Build history of the part. All positions in model axes, mm. Round coordinates to 2 decimals unless told otherwise and drop trailing zeros. Order: outer loops, then holes, each group sorted by start corner. A loop starts at its lowest first (then second) coordinate and runs counter-clockwise, first axis right, second up. Notation, with made-up numbers: (86, -35.75) - (141, -35.75) arc R33 cw to (141, -6.75) - close; hole circle Ø3 at (51, 17). An arc over 180 degrees is marked (long way). Write each question's results on one line, items separated by ' | '. Start each with the question number.
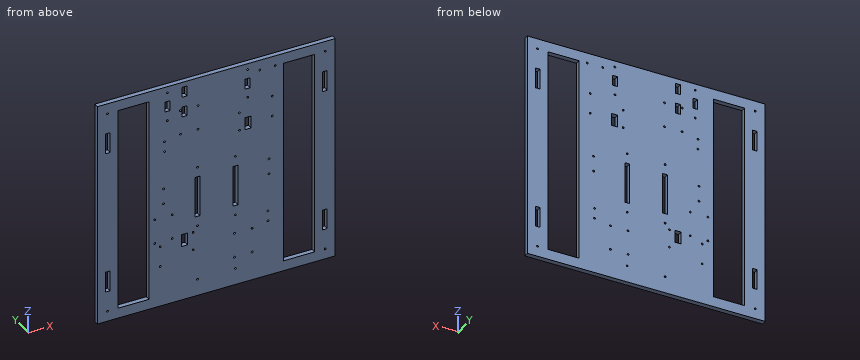
```python
from build123d import *

# Parameters (mm, degrees)
SKETCH1_W           = 292.1
SKETCH1_H           = 279.4
BOSS_EXTRUDE1_DEPTH = 5.9436
SKETCH2_W           = 38.1
SKETCH2_H           = 254
SKETCH2_W_2         = 5.9309
SKETCH2_H_2         = 25.4
CUT_EXTRUDE1_DEPTH  = 6.9436
SKETCH5_R           = 1.1303
SKETCH5_W           = 7.366
SKETCH5_H           = 15.24
CUT_EXTRUDE2_DEPTH  = 6.9436
SKETCH7_R           = 1.1303
SKETCH7_W           = 5.9436
SKETCH7_H           = 12.7
CUT_EXTRUDE3_DEPTH  = 6.9436
SKETCH9_R           = 1.1303
CUT_EXTRUDE4_DEPTH  = 6.9436
SKETCH10_W          = 5.9436
SKETCH10_H          = 50.8
CUT_EXTRUDE5_DEPTH  = 6.9436
SKETCH12_R          = 1.1303
CUT_EXTRUDE6_DEPTH  = 6.9436


with BuildPart() as part:
    # Sketch1 → Boss-Extrude1 (new body)
    with BuildSketch(Plane(origin=(0, 0, 0), x_dir=(1, 0, 0), z_dir=(0, 1, 0))):
        Rectangle(SKETCH1_W, SKETCH1_H)
    extrude(amount=BOSS_EXTRUDE1_DEPTH)

    # Sketch2 → Cut-Extrude1 (cut, through all)
    with BuildSketch(Plane(origin=(0, 5.9436, 0), x_dir=(1, 0, 0), z_dir=(0, 1, 0))):
        with Locations((-101.6, 0)):
            Rectangle(SKETCH2_W, SKETCH2_H)
        with Locations((101.6, 0)):
            Rectangle(SKETCH2_W, SKETCH2_H)
        with Locations((133.35, 88.9)):
            Rectangle(SKETCH2_W_2, SKETCH2_H_2)
        with Locations((-133.35, 88.9)):
            Rectangle(SKETCH2_W_2, SKETCH2_H_2)
        with Locations((133.35, -88.9)):
            Rectangle(SKETCH2_W_2, SKETCH2_H_2)
        with Locations((-133.35, -88.9)):
            Rectangle(SKETCH2_W_2, SKETCH2_H_2)
    extrude(amount=-CUT_EXTRUDE1_DEPTH, mode=Mode.SUBTRACT)

    # Sketch5 → Cut-Extrude2 (cut, through all)
    with BuildSketch(Plane.XZ):
        with Locations((-43.99385, 104.14)):
            Circle(SKETCH5_R)
        with Locations((-22.40385, 104.14)):
            Circle(SKETCH5_R)
        with Locations((-43.99385, 73.66)):
            Circle(SKETCH5_R)
        with Locations((-22.40385, 73.66)):
            Circle(SKETCH5_R)
        with Locations((28.37815, 79.502)):
            Circle(SKETCH5_R)
        with Locations((28.37815, 57.15)):
            Circle(SKETCH5_R)
        with Locations((68.761578288, 88.9)):
            Circle(SKETCH5_R)
        with Locations((68.761578288, 63.5)):
            Circle(SKETCH5_R)
        with Locations((-63.5, 69.85)):
            Circle(SKETCH5_R)
        with Locations((44.00655, -73.66)):
            Circle(SKETCH5_R)
        with Locations((44.00655, -104.14)):
            Circle(SKETCH5_R)
        with Locations((22.41655, -104.14)):
            Circle(SKETCH5_R)
        with Locations((22.41655, -73.66)):
            Circle(SKETCH5_R)
        with Locations((-28.36545, -79.502)):
            Circle(SKETCH5_R)
        with Locations((-28.36545, -57.15)):
            Circle(SKETCH5_R)
        with Locations((-68.748878288, -63.5)):
            Circle(SKETCH5_R)
        with Locations((-68.748878288, -88.9)):
            Circle(SKETCH5_R)
        with Locations((-63.5, 57.15)):
            Circle(SKETCH5_R)
        with Locations((63.5, -69.85)):
            Circle(SKETCH5_R)
        with Locations((63.5, -57.15)):
            Circle(SKETCH5_R)
        with Locations((-64.77, 9.627315903)):
            Circle(SKETCH5_R)
        with Locations((-64.77, -9.422684097)):
            Circle(SKETCH5_R)
        with Locations((64.77, -9.610296009)):
            Circle(SKETCH5_R)
        with Locations((64.77, 9.439703991)):
            Circle(SKETCH5_R)
        with Locations((-133.7564, -127)):
            Circle(SKETCH5_R)
        with Locations((-133.7564, 127)):
            Circle(SKETCH5_R)
        with Locations((133.7564, -127)):
            Circle(SKETCH5_R)
        with Locations((133.7564, 127)):
            Circle(SKETCH5_R)
        with Locations((39.17315, 63.5)):
            Rectangle(SKETCH5_W, SKETCH5_H)
        with Locations((-39.16045, -63.5)):
            Rectangle(SKETCH5_W, SKETCH5_H)
    extrude(amount=-CUT_EXTRUDE2_DEPTH, mode=Mode.SUBTRACT)

    # Sketch7 → Cut-Extrude3 (cut, through all)
    with BuildSketch(Plane(origin=(0, 5.9436, 0), x_dir=(1, 0, 0), z_dir=(0, 1, 0))):
        with Locations((53.410346989, -127)):
            Circle(SKETCH7_R)
        with Locations((72.460346989, -127)):
            Circle(SKETCH7_R)
        with Locations((-60.069552222, -95.996553949)):
            Circle(SKETCH7_R)
        with Locations((-60.069552222, -131.742630767)):
            Circle(SKETCH7_R)
        with Locations((38.527322113, -96.482293749)):
            Circle(SKETCH7_R)
        with Locations((38.527322113, -132.062224084)):
            Circle(SKETCH7_R)
        with Locations((-60.059259893, -114.3)):
            Rectangle(SKETCH7_W, SKETCH7_H)
        with Locations((-38.875659893, -101.6)):
            Rectangle(SKETCH7_W, SKETCH7_H)
        with Locations((-38.875659893, -127)):
            Rectangle(SKETCH7_W, SKETCH7_H)
        with Locations((38.527322113, -114.207868653)):
            Rectangle(SKETCH7_W, SKETCH7_H)
    extrude(amount=-CUT_EXTRUDE3_DEPTH, mode=Mode.SUBTRACT)

    # Sketch9 → Cut-Extrude4 (cut, through all)
    with BuildSketch(Plane(origin=(0, 5.9436, 0), x_dir=(1, 0, 0), z_dir=(0, 1, 0))):
        with Locations((23.4442, 50.154484486)):
            Circle(SKETCH9_R)
        with Locations((23.4442, 119.039284486)):
            Circle(SKETCH9_R)
        with Locations((23.4442, -25.086665514)):
            Circle(SKETCH9_R)
        with Locations((-23.1394, 119.039284486)):
            Circle(SKETCH9_R)
        with Locations((-23.1394, 50.154484486)):
            Circle(SKETCH9_R)
        with Locations((-23.1394, -25.086665514)):
            Circle(SKETCH9_R)
    extrude(amount=-CUT_EXTRUDE4_DEPTH, mode=Mode.SUBTRACT)

    # Sketch10 → Cut-Extrude5 (cut, through all)
    with BuildSketch(Plane(origin=(0, 5.9436, 0), x_dir=(1, 0, 0), z_dir=(0, 1, 0))):
        with Locations((23.4442, 12.665075)):
            Rectangle(SKETCH10_W, SKETCH10_H)
        with Locations((-23.1394, 12.665075)):
            Rectangle(SKETCH10_W, SKETCH10_H)
    extrude(amount=-CUT_EXTRUDE5_DEPTH, mode=Mode.SUBTRACT)

    # Sketch12 → Cut-Extrude6 (cut, through all)
    with BuildSketch(Plane(origin=(0, 5.9436, 0), x_dir=(1, 0, 0), z_dir=(0, 1, 0))):
        with Locations((-75.6666, 26.7462)):
            Circle(SKETCH12_R)
        with Locations((-75.6666, 57.2262)):
            Circle(SKETCH12_R)
        with Locations((-54.0766, 57.2262)):
            Circle(SKETCH12_R)
        with Locations((-54.0766, 26.7462)):
            Circle(SKETCH12_R)
    extrude(amount=-CUT_EXTRUDE6_DEPTH, mode=Mode.SUBTRACT)


solid = part.part
```
1. Flat gauge pin, fed straight in: pin 1 Ø1.5 at (x, z) = (-64.5, -105.5) entering from -Y. Where does the tip first touch, or does it go through?
2. Wall check: line 1 (Z direction, x = 63.5, y = 1.5); line 2 (X direction, y = 4.15, z = 50); line 3 (X direction, y = 3, z = -82). Give the ranges that are in metal, low to high. Write a range as from..to.
3. Cut at C-C (y = 3.4). Give the number of separate pieces and of enclosed holes in the cut face, plus the area to 3 significant figures.
4. Cut at A-A (z = 114). List the corners of the cut face in (x, y).
5. Cut at B-B (x = -96). List the corners of the cut face in (y, z).
A:
1) pin 1: stops at y = 0
2) line 1: z = -139.7..-70.98, -68.72..-58.28, -56.02..139.7 | line 2: x = -146.05..-120.65, -82.55..82.55, 120.65..146.05 | line 3: x = -146.05..-136.32, -130.38..-120.65, -82.55..82.55, 120.65..130.38, 136.32..146.05
3) separate pieces: 1 | enclosed holes: 58 | area: 60,300 mm^2
4) outline: (-146.05, 0) - (-120.65, 0) - (-120.65, 5.94) - (-146.05, 5.94) - close; (-82.55, 0) - (-63.03, 0) - (-63.03, 5.94) - (-82.55, 5.94) - close; (-57.09, 0) - (35.56, 0) - (35.56, 5.94) - (-57.09, 5.94) - close; (41.5, 0) - (82.55, 0) - (82.55, 5.94) - (41.5, 5.94) - close; (120.65, 0) - (146.05, 0) - (146.05, 5.94) - (120.65, 5.94) - close
5) outline: (0, -139.7) - (5.94, -139.7) - (5.94, -127) - (0, -127) - close; (0, 127) - (5.94, 127) - (5.94, 139.7) - (0, 139.7) - close
